The model under review builds one solid part; all positions refer to its coordinate system, in mm. A direction names the side the tool comes from. Round coordinates to 2 decimals unless told otherwise and drop trailing zeros. Loops run counter-clockwise (first coordinate to the right, second up) from the corner with the lowest first, then second, coordinate; pieces in that order, holes last. Notation, with made-up numbers: M 8,-39.75 L 27,-39.75 A18 ccw 27,-29.75 Z; hole C 69,0 d1. An arc over 180 degrees is marked long. Answer in a Markdown table with one row per item. Add a question column.
from build123d import *

# Parameters (mm, degrees)
SKETCH1_R           = 27.5
SKETCH1_R_2         = 1.6
SKETCH1_R_3         = 8
SKETCH1_R_4         = 2
BOSS_EXTRUDE1_DEPTH = 4
SKETCH2_R           = 4.25
CUT_EXTRUDE1_DEPTH  = 1.5


with BuildPart() as part:
    # Sketch1 → Boss-Extrude1 (new body)
    with BuildSketch(Plane(origin=(0, 0, 0), x_dir=(1, 0, 0), z_dir=(0, 1, 0))):
        Circle(SKETCH1_R)
        with Locations((0, 25)):
            Circle(SKETCH1_R_2, mode=Mode.SUBTRACT)
        with Locations((12.5, 21.650635095)):
            Circle(SKETCH1_R_2, mode=Mode.SUBTRACT)
        with Locations((21.650635095, 12.5)):
            Circle(SKETCH1_R_2, mode=Mode.SUBTRACT)
        with Locations((25, 0)):
            Circle(SKETCH1_R_2, mode=Mode.SUBTRACT)
        with Locations((21.650635095, -12.5)):
            Circle(SKETCH1_R_2, mode=Mode.SUBTRACT)
        with Locations((12.5, -21.650635095)):
            Circle(SKETCH1_R_2, mode=Mode.SUBTRACT)
        with Locations((0, -25)):
            Circle(SKETCH1_R_2, mode=Mode.SUBTRACT)
        with Locations((-12.5, -21.650635095)):
            Circle(SKETCH1_R_2, mode=Mode.SUBTRACT)
        with Locations((-21.650635095, -12.5)):
            Circle(SKETCH1_R_2, mode=Mode.SUBTRACT)
        with Locations((-25, 0)):
            Circle(SKETCH1_R_2, mode=Mode.SUBTRACT)
        with Locations((-21.650635095, 12.5)):
            Circle(SKETCH1_R_2, mode=Mode.SUBTRACT)
        with Locations((-12.5, 21.650635095)):
            Circle(SKETCH1_R_2, mode=Mode.SUBTRACT)
        Circle(SKETCH1_R_3, mode=Mode.SUBTRACT)
        with Locations((12.413030788, 0)):
            Circle(SKETCH1_R_4, mode=Mode.SUBTRACT)
        with Locations((-6.206515394, -10.75)):
            Circle(SKETCH1_R_4, mode=Mode.SUBTRACT)
        with Locations((-6.206515394, 10.75)):
            Circle(SKETCH1_R_4, mode=Mode.SUBTRACT)
    extrude(amount=BOSS_EXTRUDE1_DEPTH)

    # Sketch2 → Cut-Extrude1 (cut)
    with BuildSketch(Plane(origin=(0, 4, 0), x_dir=(1, 0, 0), z_dir=(0, 1, 0))):
        with Locations((-6.206515394, 10.75)):
            Circle(SKETCH2_R)
        with Locations((12.413030788, 0)):
            Circle(SKETCH2_R)
        with Locations((-6.206515394, -10.75)):
            Circle(SKETCH2_R)
    extrude(amount=-CUT_EXTRUDE1_DEPTH, mode=Mode.SUBTRACT)


solid = part.part
1. Take a section at A-A, the plane x = 6. State the section outline as (y, z) points.
2. For pin 1 Ø2 at (x, y) = (21, 1) entering from +Z; pin 2 Ø1.5 at (x, z) = (-6.5, 9) entering from +Y, all flat-tipped, find the tip position at first contact; note any pin that passes through.
3. Take a section at C-C, the plane z = 10. State the section outline as (x, y) points.
4. Mouldability with a two-part tool opening along Z and no side actions: class faces 1 (the cylindrical face through (-0.208, 1.972, 23.414)), 2 (the flat face through (6, 0, 6)), 3 (the cylindrical face through (-5.961, 1.972, 26.846)), 4 (the cylindrical face through (-13.68, 1.97, 20.57)) as released by +Z, released by -Z, zero draft, split by the parting line, or undercut.
5. Take a section at D-D, the plane y = 3.35. State how many separate pieces and enclosed holes the cut face has, and give its area (3 significant figures).
6. To check wall thickness, follow probe 1 along Z at (x, y) = (0, 2.4); probe 2 along X at (y, z) = (2, 0); probe 3 along Z at (x, y) = (-12.5, 3). State the ranges of each line that lie inside material, in increasing order.
7. Take a section at B-B, the plane z = 22.5. State the section outline as (x, y) points.
8. Machinability: for faces 5 (the cylindrical face through (-20.125, 1.972, -12.981)), 6 (the flat face through (-5, 2.5, 13)), which of the approach directions +Z, -Z, +X, -X, +Y, -Y give a long, thin tool a straight path to every point of the face, cutting with its end or side? Answer none if there is none.
Check sheet entries:
| question | item | result |
|---|---|---|
| 1 | outline | M 0,-26.84 L 4,-26.84 L 4,-5.29 L 0,-5.29 Z; M 0,5.29 L 4,5.29 L 4,26.84 L 0,26.84 Z |
| 2 | pin 1 | stops at z = 18.87 |
| 2 | pin 2 | stops at y = 2.5 |
| 3 | outline | M -25.62,0 L -8.06,0 L -8.06,2.5 L -10.39,2.5 L -10.39,4 L -25.62,4 Z; M -4.35,0 L 25.62,0 L 25.62,4 L -2.02,4 L -2.02,2.5 L -4.35,2.5 Z |
| 4 | face 1 | undercut |
| 4 | face 2 | zero draft |
| 4 | face 3 | split by the parting line |
| 4 | face 4 | undercut |
| 5 | separate pieces | 1 |
| 5 | enclosed holes | 16 |
| 5 | area | 1,910 mm^2 |
| 6 | probe 1 | z = -27.5 to -26.6, -23.4 to -8, 8 to 23.4, 26.6 to 27.5 |
| 6 | probe 2 | x = -27.5 to -26.6, -23.4 to -8, 8 to 10.41, 14.41 to 23.4, 26.6 to 27.5 |
| 6 | probe 3 | z = -24.49 to -23.25, -20.05 to 20.05, 23.25 to 24.49 |
| 7 | outline | M -15.81,0 L -13.86,0 L -13.86,4 L -15.81,4 Z; M -11.14,0 L 11.14,0 L 11.14,4 L -11.14,4 Z; M 13.86,0 L 15.81,0 L 15.81,4 L 13.86,4 Z |
| 8 | face 5 | +Y, -Y |
| 8 | face 6 | +Y |
